Autodesk Inventor part; units mm, degrees
ref_plane "YZ Plane" through (0, 0, 0) normal (1, 0, 0) x (0, 1, 0)
ref_plane "XZ Plane" through (0, 0, 0) normal (0, 1, 0) x (-1, 0, 0)
ref_plane "XY Plane" through (0, 0, 0) normal (0, 0, 1) x (1, 0, 0)
sketch "スケッチ1" plane through (0, 0, 0) normal (0, 0, 1) x (1, 0, 0)
  line L0 (-23, 23) -> (23, 23)
  line L1 (23, 23) -> (23, -23)
  line L2 (23, -23) -> (-23, -23)
  line L3 (-23, -23) -> (-23, 23)
  point P0 (0, 0)
  dimension "d0" = 46
  dimension "d1" = 46
  dimension "d2" = 23
  dimension "d3" = 23
extrude "押し出し1" add sketch "スケッチ1" along normal blind 16.5
sketch "スケッチ2" plane through (23, -23, 0) normal (1, 0, 0) x (0, 0, -1)
  line L0 (0, 0) -> (-16.5, 0)
  line L1 (0, 46) -> (-16.5, 46)
  circle A0 centre (-13.5, 38) radius 1
  circle A1 centre (-13.5, 8) radius 1
  line L2 (-16.5, 46) -> (-16.5, 0)
  point P0 (0, 23)
  dimension "d6" = 2
  dimension "d8" = 8
  dimension "d13" = 8
  dimension "d48" = 3
  dimension "d50" = 3
hole "穴1" at (23, -15, 13.5) at (23, 15, 13.5) direction (-1, 0, 0) diameter 2 end through all
sketch "スケッチ3" plane through (-23, -23, 0) normal (0, -1, 0) x (1, 0, 0)
  line L0 (46, 16.5) -> (0, 16.5)
  line L1 (0, 0) -> (0, 16.5)
  line L2 (46, 0) -> (46, 16.5)
  circle A0 centre (8, 13.5) radius 1
  circle A1 centre (38, 13.5) radius 1
  point P0 (23, 0)
  dimension "d22" = 2
  dimension "d23" = 3
  dimension "d25" = 3
  dimension "d26" = 8
  dimension "d27" = 8
hole "穴2" at (-15, -23, 13.5) at (15, -23, 13.5) direction (0, 1, 0) diameter 2 end through all
thread "ねじ1"
thread "ねじ3"
thread "ねじ5"
thread "ねじ6"
sketch "スケッチ4" plane through (0, 0, 16.5) normal (0, 0, 1) x (1, 0, 0)
  line L0 (-23, -23) -> (-23, 23)
  line L1 (23, -23) -> (-23, -23)
  circle A0 centre (-14, 19) radius 1.5
  circle A1 centre (8, 19) radius 1.5
  circle A2 centre (-14, -19) radius 1.5
  circle A3 centre (8, -19) radius 1.5
  dimension "d51" = 3
  dimension "d52" = 22
  dimension "d53" = 22
  dimension "d54" = 38
  dimension "d55" = 38
  dimension "d88" = 9
  dimension "d89" = 9
  dimension "d90" = 4
  dimension "d91" = 4
hole "穴3" at (-14, -19, 16.5) at (-14, 19, 16.5) at (8, -19, 16.5) at (8, 19, 16.5) direction (0, 0, -1) diameter 3 end through all
thread "ねじ7"
thread "ねじ8"
thread "ねじ9"
thread "ねじ10"
thread "ねじ11"
thread "ねじ13"
thread "ねじ14"
thread "ねじ16"
properties part number "14" material "アセタール樹脂、白"
Geometry check sheet. Reference: the model listing, model coordinates, mm. Give positions to 0.01 mm unless a question says otherwise; leave off trailing zeros. Order: outer loops, then holes, each group sorted by start corner. A loop starts at its lowest first (then second) coordinate and runs counter-clockwise, first axis right, second up. Notation, with made-up numbers: (-7, 11.25) - (30, 11.25) arc R25 ccw to (30, 41.25) - close; hole circle Ø10 at (30, 75). An arc over 180 degrees is marked (long way). Answer in a Markdown table with one row per item. Add a question column.
Q1. Cross-section at B-B, the plane z = 13.5. Count the separate pieces of the cut face and the enclosed holes in it, then the cut area to 3 significant figures.
Q2. Material ranges on probe 1 along Y at (x, z) = (8, 5.25); probe 2 along X at (y, z) = (-19, 8.25); probe 3 along Y at (x, z) = (-20.75, 13.5), recorded low to high. Write a range as from..to.
Q3. Cross-section at A-A, the plane y = -19. Enter the section's corners in (x, z), then the cut area to 3 significant figures.
Q4. Mould release check, pull along Z, two halves, no side actions. Record for faces 1 (the flat face through (0, 0, 0)), 2 (the cylindrical face through (-19.056, 15.383, 12.576)), 3 (the cylindrical face through (-12.67, 18.31, 8.13)): pulls with the +Z half, pulls with the -Z half, needs draft (parallel to the pull), parting line crosses it, or undercut.
Check values:
| question | item | result |
|---|---|---|
| 1 | separate pieces | 9 |
| 1 | enclosed holes | 2 |
| 1 | area | 1,740 mm^2 |
| 2 | probe 1 | y = -23..-20.5, -17.5..17.5, 20.5..23 |
| 2 | probe 2 | x = -23..-15.5, -12.5..6.5, 9.5..23 |
| 2 | probe 3 | y = -23..-16, -14..14, 16..23 |
| 3 | outline | (-23, 0) - (-15.5, 0) - (-15.5, 12.63) arc R1 cw to (-15.5, 14.37) - (-15.5, 16.5) - (-23, 16.5) - close; (-12.5, 0) - (6.5, 0) - (6.5, 16.5) - (-12.5, 16.5) - close; (9.5, 0) - (23, 0) - (23, 16.5) - (9.5, 16.5) - close; hole circle Ø2 at (15, 13.5) |
| 3 | area | 656 mm^2 |
| 4 | face 1 | pulls with the -Z half |
| 4 | face 2 | undercut |
| 4 | face 3 | needs draft |
